Could you check a few things on this drawing? It's one solid part, dimensions in mm from its lowest x, y, z. A direction names the side the tool comes from. Give positions to 0.01 mm unless a question says otherwise; leave off trailing zeros. Order: outer loops, then holes, each group sorted by start corner. A loop starts at its lowest first (then second) coordinate and runs counter-clockwise, first axis right, second up. Notation, with made-up numbers: (45, 48) -> (64, 48) arc R17 cw to (64, 80) -> close; hole circle Ø6 at (15, 26.25). An arc over 180 degrees is marked (long way). Answer as a JSON object with one key per item and string values.
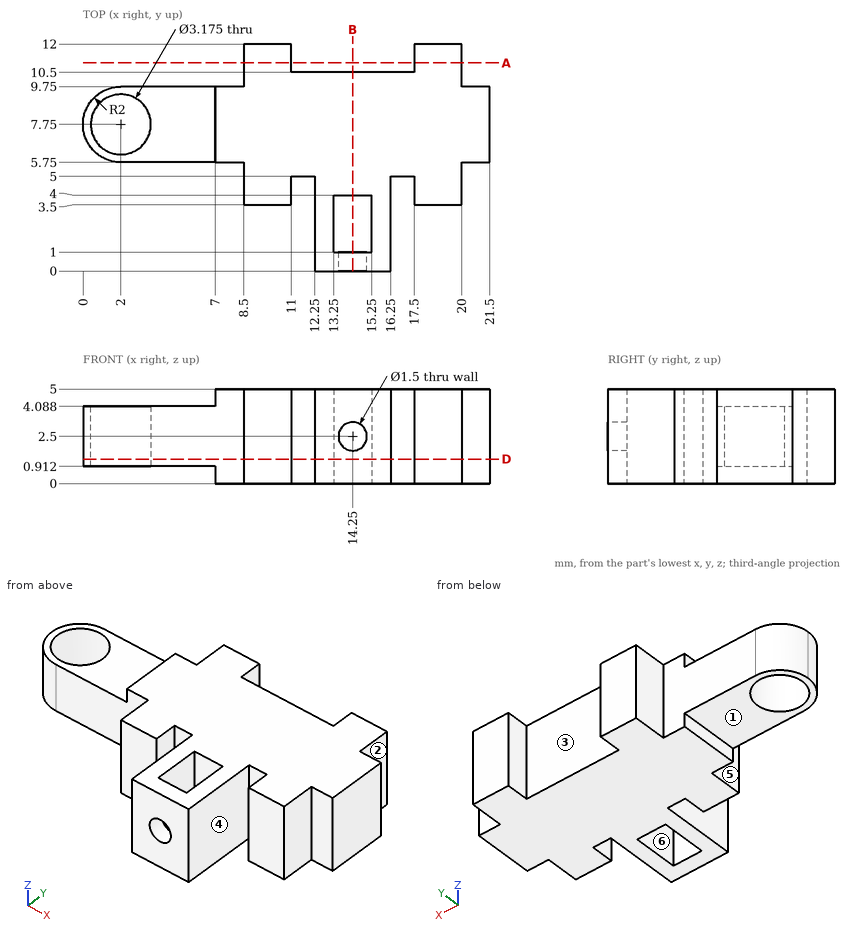
1. For the marked faces 4, 5 and 6, which set-ups out of +Z, -Z, +X, -X, +Y, -Y let a thin tool reach every point of the face, with its end or its side?
Worked answers:
{"face 4": "+Z, -Z, -Y", "face 5": "+Z, -Z, -X, -Y", "face 6": "+Z, -Z"}
2. If we mould it in two halves opening along X, with no side actions, what happens to the marked faces 1, 2 and 3? For each: +X half, -X half, draft (parallel to the pull), parting line (faces both ways), or undercut.
Worked answers:
{"face 1": "draft", "face 2": "+X half", "face 3": "undercut"}
3. Please list where these lines run through material, in increasing order: L1, parallel to X at y = 4.25, z = 3.65; L2, parallel to Z at x = 14.25, y = 0.3; L3, parallel to X at y = 5.5, z = 1.55.
Worked answers:
{"L1": "8.5 to 11, 12.25 to 16.25, 17.5 to 20", "L2": "0 to 1.75, 3.25 to 5", "L3": "8.5 to 20"}
4. If we section it at D-D on z = 1.3: Count the separate pieces of the cut face and the enclosed holes in it, then the cut area to 3 significant figures.
Worked answers:
{"separate pieces": "1", "enclosed holes": "2", "area": "123 mm²"}
5. If we section it at B-B on x = 14.25: Please give me the cut outline in (y, z), then the cut area to 3 significant figures.
Worked answers:
{"outline": "(0, 0) -> (1, 0) -> (1, 1.75) -> (0, 1.75) -> close; (0, 3.25) -> (1, 3.25) -> (1, 5) -> (0, 5) -> close; (4, 0) -> (10.5, 0) -> (10.5, 5) -> (4, 5) -> close", "area": "36.0 mm²"}
6. If we section it at A-A on y = 11: Please give me the cut outline in (x, z).
Worked answers:
{"outline": "(8.5, 0) -> (11, 0) -> (11, 5) -> (8.5, 5) -> close; (17.5, 0) -> (20, 0) -> (20, 5) -> (17.5, 5) -> close"}
7. Will these pins go through, and if not, where does the flat tip stop? pin 1 Ø4 at (x, y) = (3.5, 4.5) entering from -Z; pin 2 Ø3 at (x, z) = (9.5, 3) entering from -Y; pin 3 Ø1.5 at (y, z) = (3, 2.5) entering from +X.
Worked answers:
{"pin 1": "z = 0.91", "pin 2": "y = 3.5", "pin 3": "x = 20"}
